from build123d import *

# Parameters (mm, degrees)
F0_R     = 4.7625
F1_DEPTH = 12.7
F2_W     = 0.698456
F2_H     = 2.279171


with BuildPart() as f1:
    # F0 (on Right) → F1 (new body)
    with BuildSketch(Plane.YZ):
        Circle(F0_R)
    extrude(amount=F1_DEPTH)

    # F2 (on Top) → F3 (revolve, cut)
    with BuildSketch(Plane.XY):
        with Locations((11.419214, 4.052942)):
            Rectangle(F2_W, F2_H)
    revolve(axis=Axis((11.608969, 0, 0), (-1, 0, 0)), mode=Mode.SUBTRACT)

    # F4: F1 across plane


with BuildPart() as f1_1:
    add(f1.part)
    add(f1.part.mirror(Plane.YZ))


solid = f1_1.part
Could you check a few things on this model? Use its own coordinates, in mm. A direction names the side the tool comes from. Give positions to 0.01 mm unless a question says otherwise; leave off trailing zeros. Order: outer loops, then holes, each group sorted by start corner. A loop starts at its lowest first (then second) coordinate and runs counter-clockwise, first axis right, second up.
1. Suppose I cut it at A-A (z = 0). List the corners of the cut face in (x, y) for me, plus the area to 3 significant figures.
2. I need wall thicknesses on L1, parallel to X at y = 0.5, z = 3.25; L2, parallel to Y at x = -6.75, z = 1; L3, parallel to Z at x = 8.25, y = 3.5. Which ranges of each line are inside material? Lowest first, please.
3. Will these pins go through, and if not, where does the flat tip stop? P1, Ø1, axis at x = 4.5, y = 1.5, coming from the +Z side; P2, Ø5, axis at x = 9, z = -3.5, coming from the -Y side; P3, Ø5, axis at x = -8.5, z = 3.5, coming from the +Y side.
4. For faces 4 (the cylindrical face through (-12.23, -3.78, -2.9)), 5 (the flat face through (-11.768, 0.1, 3.1)), which set-ups out of +Z, -Z, +X, -X, +Y, -Y let a thin tool reach every point of the face, with its end or its side?
5. Suppose I cut it at B-B (y = 3.25). List the corners of the cut face in (x, z) for me.
6. We'd pull the mould along X, two halves only. Please class faces 1 (the flat face through (-12.7, 0, 0)), 2 (the flat face through (12.7, 0, 0)), 3 (the flat face through (-11.07, 0.1, 3.1)): pulls with the +X half, pulls with the -X half, needs draft (parallel to the pull), parting line crosses it, or undercut.
7. Suppose I cut it at C-C (z = 3.75). List the corners of the cut face in (x, y) for me.
Solved:
1. outline: (-12.7, -4.76) - (-11.77, -4.76) - (-11.77, -2.91) - (-11.07, -2.91) - (-11.07, -4.76) - (11.07, -4.76) - (11.07, -2.91) - (11.77, -2.91) - (11.77, -4.76) - (12.7, -4.76) - (12.7, 4.76) - (11.77, 4.76) - (11.77, 2.91) - (11.07, 2.91) - (11.07, 4.76) - (-11.07, 4.76) - (-11.07, 2.91) - (-11.77, 2.91) - (-11.77, 4.76) - (-12.7, 4.76) - close
1. area: 237 mm2
2. L1: x = -12.7 to -11.77, -11.07 to 11.07, 11.77 to 12.7
2. L2: y = -4.66 to 4.66
2. L3: z = -3.23 to 3.23
3. P1: stops at z = 4.66
3. P2: stops at y = -4.66
3. P3: stops at y = 4.66
4. face 4: +X, -X
4. face 5: none
5. outline: (-12.7, -3.48) - (-11.77, -3.48) - (-11.77, 3.48) - (-12.7, 3.48) - close; (-11.07, -3.48) - (11.07, -3.48) - (11.07, 3.48) - (-11.07, 3.48) - close; (11.77, -3.48) - (12.7, -3.48) - (12.7, 3.48) - (11.77, 3.48) - close
6. face 1: pulls with the -X half
6. face 2: pulls with the +X half
6. face 3: undercut
7. outline: (-12.7, -2.94) - (-11.77, -2.94) - (-11.77, 2.94) - (-12.7, 2.94) - close; (-11.07, -2.94) - (11.07, -2.94) - (11.07, 2.94) - (-11.07, 2.94) - close; (11.77, -2.94) - (12.7, -2.94) - (12.7, 2.94) - (11.77, 2.94) - close
